from build123d import *

# Parameters (mm, degrees)
SKETCH1_W                                            = 85
SKETCH1_H                                            = 65
BOSS_EXTRUDE1_DEPTH                                  = 8
CSK_FOR_M4_HEX_SOCKET_COUNTERSUNK_CAP_SC_D           = 4.5
CSK_FOR_M4_HEX_SOCKET_COUNTERSUNK_CAP_SC_DEPTH       = 10.648063607
CSK_FOR_M4_HEX_SOCKET_COUNTERSUNK_CAP_SC_CSINK_D     = 8.96
CSK_FOR_M4_HEX_SOCKET_COUNTERSUNK_CAP_SC_CSINK_ANGLE = 90
CSK_FOR_M4_HEX_SOCKET_COUNTERSUNK_CAP_SC_TIP         = 1.351936393
CSK_FOR_M3_HEX_SOCKET_COUNTERSUNK_CAP_SC_D           = 3.4
CSK_FOR_M3_HEX_SOCKET_COUNTERSUNK_CAP_SC_DEPTH       = 10.978536948
CSK_FOR_M3_HEX_SOCKET_COUNTERSUNK_CAP_SC_CSINK_D     = 6.72
CSK_FOR_M3_HEX_SOCKET_COUNTERSUNK_CAP_SC_CSINK_ANGLE = 90
CSK_FOR_M3_HEX_SOCKET_COUNTERSUNK_CAP_SC_TIP         = 1.021463052
SKETCH11_W                                           = 5
SKETCH11_H                                           = 65
CUT_EXTRUDE1_DEPTH                                   = 108.30330843
FILLET1_R                                            = 20


with BuildPart() as part:
    # Sketch1 → Boss-Extrude1 (new body)
    with BuildSketch(Plane.XY):
        with Locations((42.5, 32.5)):
            Rectangle(SKETCH1_W, SKETCH1_H)
    extrude(amount=BOSS_EXTRUDE1_DEPTH)

    # CSK for M4 Hex Socket Countersunk Cap Screw1
    with Locations(Plane(origin=(0, 0, 0), x_dir=(-1, 0, 0), z_dir=(0, 0, -1))):
        with Locations((-70, 57.5), (-20, 57.5), (-20, 32.5), (-70, 32.5), (-70, 7.5), (-20, 7.5)):
            CounterSinkHole(CSK_FOR_M4_HEX_SOCKET_COUNTERSUNK_CAP_SC_D / 2, CSK_FOR_M4_HEX_SOCKET_COUNTERSUNK_CAP_SC_CSINK_D / 2, depth=CSK_FOR_M4_HEX_SOCKET_COUNTERSUNK_CAP_SC_DEPTH, counter_sink_angle=CSK_FOR_M4_HEX_SOCKET_COUNTERSUNK_CAP_SC_CSINK_ANGLE)
            with Locations((0, 0, -(CSK_FOR_M4_HEX_SOCKET_COUNTERSUNK_CAP_SC_DEPTH + CSK_FOR_M4_HEX_SOCKET_COUNTERSUNK_CAP_SC_TIP / 2))):  # 118° drill point
                Cone(0, CSK_FOR_M4_HEX_SOCKET_COUNTERSUNK_CAP_SC_D / 2, CSK_FOR_M4_HEX_SOCKET_COUNTERSUNK_CAP_SC_TIP, mode=Mode.SUBTRACT)

    # CSK for M3 Hex Socket Countersunk Cap Screw1
    with Locations(Plane.XY.offset(8)):
        with Locations((11, 44.728312208), (79, 44.728312208), (79, 22.728312208), (9.7, 16.028312208)):
            CounterSinkHole(CSK_FOR_M3_HEX_SOCKET_COUNTERSUNK_CAP_SC_D / 2, CSK_FOR_M3_HEX_SOCKET_COUNTERSUNK_CAP_SC_CSINK_D / 2, depth=CSK_FOR_M3_HEX_SOCKET_COUNTERSUNK_CAP_SC_DEPTH, counter_sink_angle=CSK_FOR_M3_HEX_SOCKET_COUNTERSUNK_CAP_SC_CSINK_ANGLE)
            with Locations((0, 0, -(CSK_FOR_M3_HEX_SOCKET_COUNTERSUNK_CAP_SC_DEPTH + CSK_FOR_M3_HEX_SOCKET_COUNTERSUNK_CAP_SC_TIP / 2))):  # 118° drill point
                Cone(0, CSK_FOR_M3_HEX_SOCKET_COUNTERSUNK_CAP_SC_D / 2, CSK_FOR_M3_HEX_SOCKET_COUNTERSUNK_CAP_SC_TIP, mode=Mode.SUBTRACT)

    # Sketch11 → Cut-Extrude1 (cut, through all)
    with BuildSketch(Plane.XY.offset(8)):
        with Locations((2.5, 32.5)):
            Rectangle(SKETCH11_W, SKETCH11_H)
    extrude(amount=-CUT_EXTRUDE1_DEPTH, mode=Mode.SUBTRACT)

    # Fillet1
    fillet1_edges = [part.edges().sort_by_distance(p)[0] for p in [
        (85, 65, 4),
        (85, 0, 4),
        (5, 65, 4),
        (5, 0, 4),
    ]]
    fillet(fillet1_edges, radius=FILLET1_R)


solid = part.part
Work out the finished part from the listing and answer in its coordinate system (mm). Coordinates: 2 decimals unless noted, no trailing zeros. Write each loop counter-clockwise with the first axis right and the second up, starting at its lowest first coordinate (ties: lowest second). Pieces come first, ordered by that corner, then holes. Notation, with made-up numbers: M 24.5,46 L 57.5,46 A16 cw 57.5,59 Z; hole C 27,-19.75 d6. An arc over 180 degrees is marked long. Answer as CSV lines item,"result". Start each with the question number.
Item 1: Consider L1, parallel to X at y = 32.5, z = 6; L2, parallel to Y at x = 69.5, z = 7.75; L3, parallel to X at y = 7.5, z = 6.8. Determine where each line is inside the solid, lowest interval first.
Item 2: Flat-ended cylindrical pins translate along their axes: P1, Ø5, axis at x = 70, y = 57.5, coming from the +Z side; P2, Ø5.5, axis at x = 9.7, y = 16.03, coming from the +Z side; P3, Ø3, axis at x = 73.5, z = 3.5, coming from the +Y side (3 decimals); P4, Ø4, axis at y = 50, z = 2, coming from the -X side. Find the tip coordinate at first contact, or state that the pin passes through.
Item 3: Determine the mould class of faces 1 (the face through (10.703, 58.986, 3.944)), 2 (the face through (71.21, 9.397, 5.155)), 3 (the face through (5, 32, 4)), 4 (the face through (80.7, 22.8, 3.1)) for opening direction Y: released by +Y, released by -Y, zero draft, split by the parting line, or undercut.
Item 4: Section C-C on x = 79 is taken. Write down the section's boundary in (y, z).
Item 5: Section A-A on y = 32.5 is taken. Write down the section's boundary in (x, z), and give its area (3 significant figures).
Item 6: Section B-B on x = 20 is taken. Write down the section's boundary in (y, z).
Item 7: Section D-D on z = 5 is taken. Give the number of separate pieces and of enclosed holes in the cut face, and give its area (3 significant figures).
Checks:
1,L1,"x = 5 to 17.75, 22.25 to 67.75, 72.25 to 85"
1,L2,"y = 0.51 to 5.31, 9.69 to 30.31, 34.69 to 55.31, 59.69 to 64.49"
1,L3,"x = 9.39 to 17.75, 22.25 to 67.75, 72.25 to 80.61"
2,P1,"stops at z = 8"
2,P2,"stops at z = 7.39"
2,P3,"stops at y = 63.735"
2,P4,"stops at x = 5.23"
3,face 1,"released by +Y"
3,face 2,"undercut"
3,face 3,"zero draft"
3,face 4,"undercut"
4,outline,"M 5.72,0 L 21.03,0 L 21.03,6.34 L 19.37,8 L 5.72,8 Z; M 24.43,0 L 43.03,0 L 43.03,6.34 L 41.37,8 L 26.09,8 L 24.43,6.34 Z; M 46.43,0 L 59.28,0 L 59.28,8 L 48.09,8 L 46.43,6.34 Z"
5,outline,"M 5,0 L 15.52,0 L 17.75,2.23 L 17.75,8 L 5,8 Z; M 22.25,2.23 L 24.48,0 L 65.52,0 L 67.75,2.23 L 67.75,8 L 22.25,8 Z; M 72.25,2.23 L 74.48,0 L 85,0 L 85,8 L 72.25,8 Z"
5,area,"558 mm²"
6,outline,"M 0.64,0 L 3.02,0 L 5.25,2.23 L 5.25,8 L 0.64,8 Z; M 9.75,2.23 L 11.98,0 L 28.02,0 L 30.25,2.23 L 30.25,8 L 9.75,8 Z; M 34.75,2.23 L 36.98,0 L 53.02,0 L 55.25,2.23 L 55.25,8 L 34.75,8 Z; M 59.75,2.23 L 61.98,0 L 64.36,0 L 64.36,8 L 59.75,8 Z"
7,separate pieces,"1"
7,enclosed holes,"10"
7,area,"4,720 mm²"
